Verification items for the finished model (mm, model axes). A direction names the side the tool comes from. Give positions to 0.01 mm unless a question says otherwise; leave off trailing zeros. Write each loop counter-clockwise with the first axis right and the second up, starting at its lowest first coordinate (ties: lowest second). Pieces come first, ordered by that corner, then holes. Notation, with made-up numbers: (57, -29) - (84, -29) arc R13 cw to (84, -25) - close; hole circle Ø1 at (53.5, -10.75). An arc over 180 degrees is marked (long way). Answer as a JSON object with one key per item and string values. Group by question number.
Item 1: Tool access check on faces 1 (the face through (4, 7, 20)), 2 (the face through (-6.944, -5.324, 9.367)). Record the directions out of +Z, -Z, +X, -X, +Y, -Y that give a thin tool (end or side, any length) a straight path to the whole face; none if there is none.
Item 2: Go/stop test with flat-tipped pins: pin 1 (1.5 mm diameter, centred on x = -6, z = 5, fed in from -Y); pin 2 (6 mm diameter, centred on x = -4.5, z = 7, fed in from -Y); pin 3 (5 mm diameter, centred on x = -4.5, z = 12.5, fed in from -Y). Record where each tip stops, or that it passes through.
Item 3: Sectioned sample at C-C, the plane z = 8.25. Record the boundary of the cut face in (x, y), and give its area (3 significant figures).
Item 4: Scan lines: line 1 along Y through (x, z) = (0, 19.75); line 2 along Y through (x, z) = (-0.25, 5.5); line 3 along X through (y, z) = (5, 13.75). Record each from-to range of solid material in increasing order. Write a range as [from, to].
Item 5: Sectioned sample at A-A, the plane x = 0. Record the boundary of the cut face in (y, z).
```python
from build123d import *

# Parameters (mm, degrees)
F0_R     = 8.75
F1_DEPTH = 19
F2_T     = -1.25
F3_R     = 10
F4_DEPTH = 1
F5_R     = 7.5
F6_DEPTH = 1.001


with BuildPart() as f1:
    # F0 (on Top) → F1 (new body)
    with BuildSketch(Plane.XY):
        Circle(F0_R)
    extrude(amount=F1_DEPTH)

    # F2
    f2_openings = [f1.faces().sort_by_distance(p)[0] for p in [
        (0, 0, 19),
        (0, 0, 0),
    ]]
    offset(amount=F2_T, openings=f2_openings)

    # F3 (on face) → F4 (join)
    with BuildSketch(Plane.XY.offset(19)):
        Circle(F3_R)
    extrude(amount=F4_DEPTH)

    # F5 (on face) → F6 (cut, through all)
    with BuildSketch(Plane(origin=(0, 0, 19), x_dir=(1, 0, 0), z_dir=(0, 0, -1))):
        Circle(F5_R)
    extrude(amount=-F6_DEPTH, mode=Mode.SUBTRACT)


solid = f1.part
```
Geometry check:
{
 "1": {"face 1": "+Z, +X, -X, +Y, -Y", "face 2": "-Z"},
 "2": {"pin 1": "y = -7", "pin 2": "y = -8.62", "pin 3": "y = -8.52"},
 "3": {"outline": "circle Ø17.5 at (0, 0); hole circle Ø15 at (0, 0)", "area": "63.8 mm^2"},
 "4": {"line 1": "[-10, -7.5], [7.5, 10]", "line 2": "[-8.75, -7.5], [7.5, 8.75]", "line 3": "[-7.18, -5.59], [5.59, 7.18]"},
 "5": {"outline": "(-10, 19) - (-8.75, 19) - (-8.75, 0) - (-7.5, 0) - (-7.5, 20) - (-10, 20) - close; (7.5, 0) - (8.75, 0) - (8.75, 19) - (10, 19) - (10, 20) - (7.5, 20) - close"}
}
